Autodesk Inventor part; units mm, degrees
ref_plane "YZ Plane" through (0, 0, 0) normal (1, 0, 0) x (0, 1, 0)
ref_plane "XZ Plane" through (0, 0, 0) normal (0, 1, 0) x (-1, 0, 0)
ref_plane "XY Plane" through (0, 0, 0) normal (0, 0, 1) x (1, 0, 0)
sketch "Sketch1" plane through (0, 0, 0) normal (0, 1, 0) x (-1, 0, 0)
  line L0 (0, 0) -> (-105.445, 0) construction
  line L1 (0, 4) -> (-105.445, 4)
  line L2 (-105.445, -4) -> (0, -4)
  arc A0 (0, -4) -> (0, 4) centre (0, 0) ccw
  arc A1 (-105.445, 4) -> (-105.445, -4) centre (-105.445, 0) ccw
  circle A2 centre (0, 0) radius 2.1
  circle A3 centre (-81.271, 0) radius 2.1
  circle A4 centre (-105.445, 0) radius 2.1
  point P0 (-52.7225, 0)
  point P1 (-52.7225, 0)
  dimension "d0" = 105.445
  dimension "d1" = 8
  dimension "d2" = 4.2
  dimension "d8" = 4.2
  dimension "d9" = 81.271
  dimension "d10" = 4.2
extrude "Extrusion1" add sketch "Sketch1" along normal blind 5
sketch "Sketch2" plane through (0, 5, 0) normal (0, 1, 0) x (1, 0, 0)
  arc A0 (105.445, -4) -> (105.445, 4) centre (105.445, 0) ccw
  line L0 (105.445, 4) -> (0, 4)
  arc A1 (0, 4) -> (0, -4) centre (0, 0) ccw
  line L1 (0, -4) -> (105.445, -4)
  circle A2 centre (81.271, 0) radius 2.1
  circle A3 centre (105.445, 0) radius 2.1
  circle A4 centre (0, 0) radius 2.1
  circle A5 centre (8, 0) radius 4
  line L2 (0, -4) -> (105.445, -4)
  circle A6 centre (97.445, 0) radius 4
  circle A7 centre (81.271, 0) radius 4
  point P0 (97.445, -4)
  point P1 (97.445, 4)
  point P2 (8, -4)
  point P3 (8, 4)
  dimension "d11" = 8
  dimension "d12" = 8
  dimension "d13" = 8
  dimension "d28" = 8
extrude "Extrusion7" add sketch "Sketch2" along normal blind 5 contours A7 | L1 A1 L0 A5 | A5
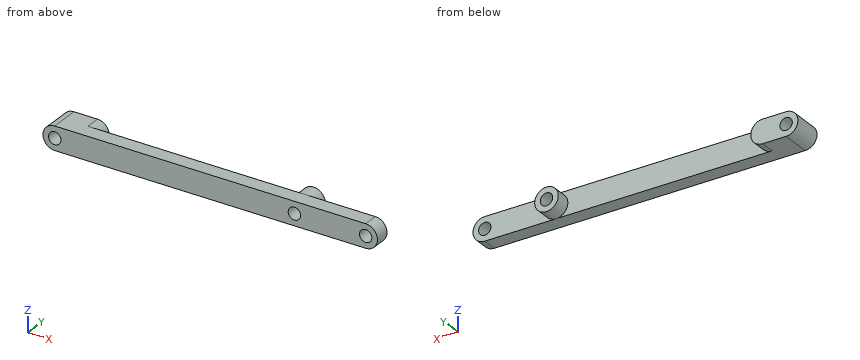
Model file for the job. Use its own axes, mm. Give positions to 0.01 mm unless a question says otherwise; leave off trailing zeros. Write each loop counter-clockwise with the first axis right and the second up, starting at its lowest first coordinate (ties: lowest second). Pieces come first, ordered by that corner, then holes. Notation, with made-up numbers: M 70.5,82.5 L 100.5,82.5 A19 cw 100.5,100.5 Z; hole C 87.5,31.5 d6. An arc over 180 degrees is marked long. One line per item, written item: value. Start each with the question number.
Q1. Saw through at B-B, the plane y = 1.5. Write the cut outline in (x, z) (3 decimals), plus the area to 3 significant figures.
Q2. Probe probe 1 along X at (y, z) = (7.75, 0); probe 2 along Z at (x, y) = (81, 5); probe 3 along Y at (x, z) = (30, -1). List the from-to ranges inside material, lowest first. Write a range as [from, to].
Q3. Saw through at C-C, the plane x = 11. Write the cut outline in (y, z), plus the area to 3 significant figures.
Q4. Saw through at A-A, the plane y = 8. Write the cut outline in (x, z), plus the area to 3 significant figures.
Q5. Saw through at D-D, the plane x = 38.5. Write the cut outline in (y, z), plus the area to 3 significant figures.
Q6. Drop a flat-ended pin along its axis: pin 1 Ø1 at (y, z) = (5, -1) entering from +X. Give the stop position or say it passes through.
Output values:
1. outline: M 0,-4 L 105.445,-4 A4 ccw 105.445,4 L 0,4 A4 ccw Z; hole C 0,0 d4.2; hole C 81.271,0 d4.2; hole C 105.445,0 d4.2
1. area: 852 mm²
2. probe 1: x = [-4, -2.1], [2.1, 12], [77.27, 79.17], [83.37, 85.27]
2. probe 2: z = [-3.99, -2.08], [2.08, 3.99]
2. probe 3: y = [0, 5]
3. outline: M 0,-4 L 5,-4 L 5,-2.65 L 10,-2.65 L 10,2.65 L 5,2.65 L 5,4 L 0,4 Z
3. area: 66.5 mm²
4. outline: M 0,-4 L 8,-4 A4 ccw 8,4 L 0,4 A4 ccw Z; C 81.27,0 d8; hole C 0,0 d4.2; hole C 81.27,0 d4.2
4. area: 137 mm²
5. outline: M 0,-4 L 5,-4 L 5,4 L 0,4 Z
5. area: 40.0 mm²
6. pin 1: stops at x = 109.41
